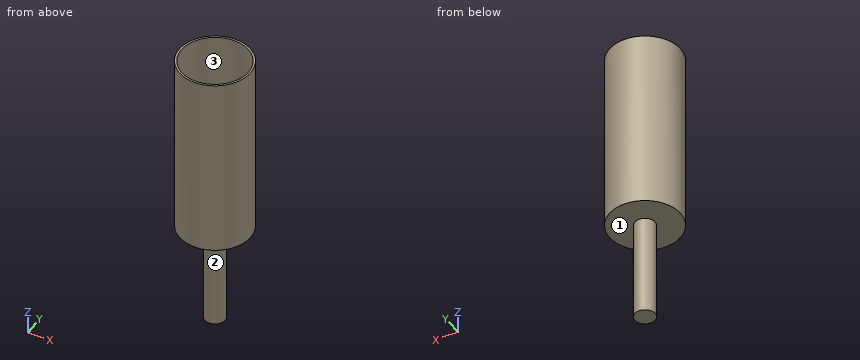
```python
from build123d import *

# Parameters (mm, degrees)
SCHIZZO1_R                   = 17.5
ESTRUSIONE_ESTRUSIONE1_DEPTH = 90
SCHIZZO2_R                   = 16.5
TAGLIO_ESTRUSIONE1_DEPTH     = 88
SCHIZZO3_R                   = 5
ESTRUSIONE_ESTRUSIONE2_DEPTH = 50


with BuildPart() as part:
    # Schizzo1 → Estrusione-Estrusione1 (new body)
    with BuildSketch(Plane.XY):
        with Locations(Location((0, 0, 0), (0, 0, 180))):
            Circle(SCHIZZO1_R)
    extrude(amount=ESTRUSIONE_ESTRUSIONE1_DEPTH)

    # Schizzo2 → Taglio-Estrusione1 (cut)
    with BuildSketch(Plane.XY.offset(90)):
        Circle(SCHIZZO2_R)
    extrude(amount=-TAGLIO_ESTRUSIONE1_DEPTH, mode=Mode.SUBTRACT)

    # Schizzo3 → Estrusione-Estrusione2 (add)
    with BuildSketch(Plane(origin=(0, 0, 0), x_dir=(-1, 0, 0), z_dir=(0, 0, -1))):
        Circle(SCHIZZO3_R)
    extrude(amount=ESTRUSIONE_ESTRUSIONE2_DEPTH)


solid = part.part
```
Can you work these out from the model? Positions are in its coordinate system, mm. Face numbers are marked on the shaded views. Give positions to 0.01 mm unless a question says otherwise; leave off trailing zeros. Write each loop counter-clockwise with the first axis right and the second up, starting at its lowest first coordinate (ties: lowest second). Pieces come first, ordered by that corner, then holes. Notation, with made-up numbers: (-26, 69.25) -> (-5, 69.25) arc R32 ccw to (-5, 104.25) -> close; hole circle Ø6 at (65, 1). An arc over 180 degrees is marked (long way). One line per item, written item: value.
Q1. Imagine slicing it at A-A on y = 0. Please give me the cut outline in (x, z), and give its area (3 significant figures).
Results found:
outline: (-17.5, 0) -> (-5, 0) -> (-5, -50) -> (5, -50) -> (5, 0) -> (17.5, 0) -> (17.5, 90) -> (16.5, 90) -> (16.5, 2) -> (-16.5, 2) -> (-16.5, 90) -> (-17.5, 90) -> close
area: 746 mm^2
Q2. We'd pull the mould along Y, two halves only. Please class the marked faces 1, 2 and 3: +Y half, -Y half, draft (parallel to the pull), parting line (faces both ways), or undercut.
Results found:
face 1: draft
face 2: parting line
face 3: undercut
Q3. Imagine slicing it at C-C on z = 80. Please give me the cut outline in (x, y), and give its area (3 significant figures).
Results found:
outline: circle Ø35 at (0, 0); hole circle Ø33 at (0, 0)
area: 107 mm^2
Q4. Please list where these lines run through material, in increasing order: line 1 (Y direction, x = 0, z = 55.5); line 2 (Z direction, x = 1, y = 5); line 3 (X direction, y = -5.5, z = 3). Write a range as [from, to].
Results found:
line 1: y = [-17.5, -16.5], [16.5, 17.5]
line 2: z = [0, 2]
line 3: x = [-16.61, -15.56], [15.56, 16.61]
Q5. For P1, Ø1, axis at x = 3.5, y = -6.5, coming from the -Z side; P2, Ø6, axis at y = 7.5, z = 22.5, coming from the -X side; P3, Ø2, axis at x = 8, y = -1.5, coming from the +Z side, each with a flat end and sliding along its axis, tell me the tip position at first contact or that it passes through.
Results found:
P1: stops at z = 0
P2: stops at x = -16.91
P3: stops at z = 2
Q6. Imagine slicing it at D-D on y = 7. Please give me the cut outline in (x, z), and give its area (3 significant figures).
Results found:
outline: (-16.04, 0) -> (16.04, 0) -> (16.04, 90) -> (14.94, 90) -> (14.94, 2) -> (-14.94, 2) -> (-14.94, 90) -> (-16.04, 90) -> close
area: 257 mm^2
